```python
from build123d import *

# Parameters (mm, degrees)
SKETCH1_R                = 1.55
SKETCH1_R_2              = 7
SKETCH1_R_3              = 2.5
BOSS_EXTRUDE1_DEPTH      = 20
BOSS_EXTRUDE2_REACH      = 53.813
BOSS_EXTRUDE2_END_RADIUS = 18.9
BOSS_EXTRUDE3_REACH      = 55.526
BOSS_EXTRUDE3_END_RADIUS = 18.9
SKETCH3_W                = 6
SKETCH3_H                = 20
SKETCH5_R                = 1.675
CUT_EXTRUDE3_DEPTH       = 22.5
CUT_EXTRUDE4_DEPTH       = 11
CUT_EXTRUDE5_DEPTH       = 5.25
SKETCH8_R                = 1.06
CUT_EXTRUDE6_DEPTH       = 54.525694884
SKETCH9_R                = 3
CUT_EXTRUDE7_DEPTH       = 10
SKETCH11_R               = 11.2
CUT_EXTRUDE9_DEPTH       = 2.35
CUT_EXTRUDE8_DEPTH       = 6


with BuildPart() as part:
    # Sketch1 → Boss-Extrude1 (new body)
    with BuildSketch(Plane(origin=(0, 0, 0), x_dir=(1, 0, 0), z_dir=(0, 1, 0))):
        with BuildLine():
            Line((10.349494937, -15.814485593), (10.349494937, 8.416255239))
            ThreePointArc((10.349494937, 8.416255239), (10.822804202, 11.144484896), (8.349494937, 9.899494937))
            Line((8.349494937, 9.899494937), (8.349494937, -16.955705067))
            ThreePointArc((8.349494937, -16.955705067), (-17.76919177, 6.439396233), (17.273666667, 7.670100383))
            ThreePointArc((17.273666667, 7.670100383), (23, 0), (17.273666667, -7.670100383))
            ThreePointArc((17.273666667, -7.670100383), (14.399392933, -12.242037541), (10.349494937, -15.814485593))
        make_face()
        with Locations(Location((-9.899494937, 9.899494937, 0), (0, 0, 270))):
            Circle(SKETCH1_R, mode=Mode.SUBTRACT)
        with Locations(Location((-9.899494937, -9.899494937, 0), (0, 0, 270))):
            Circle(SKETCH1_R, mode=Mode.SUBTRACT)
        with Locations(Location((0, 0, 0), (0, 0, 270))):
            Circle(SKETCH1_R_2, mode=Mode.SUBTRACT)
        with Locations(Location((15, 0, 0), (0, 0, 270))):
            Circle(SKETCH1_R_3, mode=Mode.SUBTRACT)
    extrude(amount=BOSS_EXTRUDE1_DEPTH)

    # Boss-Extrude2: up to this cylinder (the profile starts outside it)
    boss_extrude2_end = Plane(origin=(0, 6.495191, 0), z_dir=(0, -1, 0)) * Cylinder(BOSS_EXTRUDE2_END_RADIUS, 146.426, mode=Mode.PRIVATE)
    # Sketch2 → Boss-Extrude2 (add, up to the surface)
    with BuildSketch(Plane.XY.offset(-23), mode=Mode.PRIVATE) as boss_extrude2_sk1:
        Polygon((14.1, 6.495190528), (10.35, 0), (2.85, 0), (-0.9, 6.495190528), (2.85, 12.990381057), (10.35, 12.990381057), align=None)
    boss_extrude2_tool1 = extrude(boss_extrude2_sk1.sketch, amount=BOSS_EXTRUDE2_REACH, mode=Mode.PRIVATE) - boss_extrude2_end
    add(boss_extrude2_tool1.solids().sort_by_distance((6.6, 6.495191, -23))[0])

    # Boss-Extrude3: up to this cylinder (the profile starts outside it)
    boss_extrude3_end = Plane(origin=(0, 9.928375, 0), z_dir=(0, -1, 0)) * Cylinder(BOSS_EXTRUDE3_END_RADIUS, 149.99525, mode=Mode.PRIVATE)
    # Sketch3 → Boss-Extrude3 (add, up to the surface)
    with BuildSketch(Plane.XY.offset(21), mode=Mode.PRIVATE) as boss_extrude3_sk1:
        with BuildLine():
            Line((8.349494937, 20), (3.349494937, 20))
            Line((3.349494937, 20), (3.349494937, 8.936698586))
            ThreePointArc((3.349494937, 8.936698586), (2.099494937, 6.5), (3.349494937, 4.063301414))
            Line((3.349494937, 4.063301414), (3.349494937, 0))
            Line((3.349494937, 0), (8.349494937, 0))
            Line((8.349494937, 0), (8.349494937, 20))
        make_face()
    boss_extrude3_tool1 = extrude(boss_extrude3_sk1.sketch, amount=-BOSS_EXTRUDE3_REACH, mode=Mode.PRIVATE) - boss_extrude3_end
    add(boss_extrude3_tool1.solids().sort_by_distance((5.726294, 9.85675, 21))[0])
    # Sketch3 → Boss-Extrude3 (add, up to the surface)
    with BuildSketch(Plane.XY.offset(21), mode=Mode.PRIVATE) as boss_extrude3_sk2:
        with Locations((13.349494937, 10)):
            Rectangle(SKETCH3_W, SKETCH3_H)
    boss_extrude3_tool2 = extrude(boss_extrude3_sk2.sketch, amount=-BOSS_EXTRUDE3_REACH, mode=Mode.PRIVATE) - boss_extrude3_end
    add(boss_extrude3_tool2.solids().sort_by_distance((13.349495, 10, 21))[0])

    # Sketch5 → Cut-Extrude3 (cut)
    with BuildSketch(Plane(origin=(16.349494937, 0, 0), x_dir=(0, 0, -1), z_dir=(1, 0, 0))):
        with Locations(Location((-17, 12, 0), (0, 0, 90))):
            Circle(SKETCH5_R)
    extrude(amount=-CUT_EXTRUDE3_DEPTH, mode=Mode.SUBTRACT)

    # Sketch6 → Cut-Extrude4 (cut)
    with BuildSketch(Plane(origin=(-6.150505063, 0, 0), x_dir=(0, 0, -1), z_dir=(1, 0, 0))):
        Polygon((-20.35, 12), (-18.675, 9.098814897), (-15.325, 9.098814897), (-13.65, 12), (-15.325, 14.901185103), (-18.675, 14.901185103), align=None)
    extrude(amount=CUT_EXTRUDE4_DEPTH, mode=Mode.SUBTRACT)

    # Sketch7 → Cut-Extrude5 (cut)
    with BuildSketch(Plane(origin=(0, 4.25, 0), x_dir=(1, 0, 0), z_dir=(0, 1, 0))):
        with BuildLine():
            Line((6.29798001, 4), (5.744562647, 4))
            Line((5.744562647, 4), (5.744562647, -4))
            Line((5.744562647, -4), (6.29798001, -4))
            ThreePointArc((6.29798001, -4), (24.577324882, 0), (6.29798001, 4))
        make_face()
    extrude(amount=CUT_EXTRUDE5_DEPTH, mode=Mode.SUBTRACT)

    # Sketch8 → Cut-Extrude6 (cut, through all)
    with BuildSketch(Plane(origin=(0, 0, -23), x_dir=(-1, 0, 0), z_dir=(0, 0, -1))):
        with Locations((-6.6, 6.495190528)):
            Circle(SKETCH8_R)
    extrude(amount=-CUT_EXTRUDE6_DEPTH, mode=Mode.SUBTRACT)

    # Sketch9 → Cut-Extrude7 (cut)
    with BuildSketch(Plane(origin=(0, 0, -23), x_dir=(-1, 0, 0), z_dir=(0, 0, -1))):
        with Locations((-6.6, 6.495190528)):
            Circle(SKETCH9_R)
    extrude(amount=-CUT_EXTRUDE7_DEPTH, mode=Mode.SUBTRACT)

    # Sketch11 → Cut-Extrude9 (cut)
    with BuildSketch(Plane(origin=(0, 20, 0), x_dir=(1, 0, 0), z_dir=(0, 1, 0))):
        Circle(SKETCH11_R)
    extrude(amount=-CUT_EXTRUDE9_DEPTH, mode=Mode.SUBTRACT)

    # Sketch10 → Cut-Extrude8 (cut)
    with BuildSketch(Plane(origin=(0, 20, 0), x_dir=(1, 0, 0), z_dir=(0, 1, 0))):
        Polygon((15, 4.7), (10.929680602, 2.35), (10.349494937, 2.35), (10.349494937, -2.35), (10.929680602, -2.35), (15, -4.7), (19.070319398, -2.35), (19.070319398, 2.35), align=None)
    extrude(amount=-CUT_EXTRUDE8_DEPTH, mode=Mode.SUBTRACT)

    # Cut-Revolve1: read off the stored shape, not the designer's step
    # Cut-Revolve1: loft between two sections, ruled curve by curve
    cut_revolve1_from = [
        Edge.make_three_point_arc((7.653578644, 6.608263478, -9.001288479), (6.491231459, 7.554083708, -9.001288479), (5.545411229, 6.391736522, -9.001288479)),
        Edge.make_three_point_arc((5.545411229, 6.391736522, -9.001288479), (6.707758415, 5.445916292, -9.001288479), (7.653578644, 6.608263478, -9.001288479)),
    ]
    cut_revolve1_to = [
        Edge.make_three_point_arc((9.086412031, 6.755427811, -4), (6.344067126, 8.986917094, -4), (4.112577842, 6.244572189, -4)),
        Edge.make_three_point_arc((4.112577842, 6.244572189, -4), (6.854922748, 4.013082906, -4), (9.086412031, 6.755427811, -4)),
    ]
    cut_revolve1 = Solid(Shell([*[Face.make_surface_from_curves(cut_revolve1_from[k], cut_revolve1_to[k]) for k in range(2)], Face(Wire(cut_revolve1_from)), Face(Wire(cut_revolve1_to))]))
    add(cut_revolve1, mode=Mode.SUBTRACT)


solid = part.part
```
Input: part model. Units: mm. Frame: model coordinates. A direction names the side the tool comes from. Round coordinates to 2 decimals unless told otherwise and drop trailing zeros. Loops run counter-clockwise (first coordinate to the right, second up) from the corner with the lowest first, then second, coordinate; pieces in that order, holes last. Notation, with made-up numbers: (-30, 36.25) -> (7, 36.25) arc R30 ccw to (7, 59.25) -> close; hole circle Ø8 at (-13.75, 4). An arc over 180 degrees is marked (long way). Write each question's results on one line, items separated by ' | '.
1. First-contact query: P1, Ø3, axis at x = -9.9, z = -9.9, coming from the +Y side; P2, Ø8, axis at x = -2.5, y = 8.5, coming from the +Z side; P3, Ø6, axis at y = 5, z = 3.5, coming from the -X side; P4, Ø1, axis at y = 12, z = -17, coming from the -X side. Flat tips, straight axial feed; report the tip coordinate or a pass-through.
Geometry results:
P1: through | P2: z = 18.9 | P3: x = -18.89 | P4: x = -9.22
2. Section B-B (x = 0). Return loops of the section in (y, z) (3 decimals).
Geometry results:
outline: (0, -18.9) -> (4.936, -18.9) -> (4.936, -23) -> (8.054, -23) -> (8.054, -18.9) -> (20, -18.9) -> (20, -11.2) -> (17.65, -11.2) -> (17.65, -7) -> (0, -7) -> close; (0, 7) -> (17.65, 7) -> (17.65, 11.2) -> (20, 11.2) -> (20, 18.9) -> (14.511, 18.9) -> (14.901, 18.675) -> (14.901, 15.325) -> (12, 13.65) -> (9.099, 15.325) -> (9.099, 18.675) -> (9.489, 18.9) -> (0, 18.9) -> close
3. Section A-A (z = 17). Return loops of the section in (x, y) (1 decimal), and give its area (3 significant figures).
Geometry results:
outline: (-8.3, 0) -> (8.3, 0) -> (8.3, 10.3) -> (4.8, 10.3) -> (4.8, 9.1) -> (-6.2, 9.1) -> (-6.2, 14.9) -> (4.8, 14.9) -> (4.8, 13.7) -> (8.3, 13.7) -> (8.3, 20) -> (-8.3, 20) -> close; (10.3, 0) -> (16.3, 0) -> (16.3, 10.3) -> (10.3, 10.3) -> close; (10.3, 13.7) -> (16.3, 13.7) -> (16.3, 20) -> (10.3, 20) -> close; hole circle Ø2.1 at (6.6, 6.5) | area: 353 mm2
4. Section D-D (x = 13.5). Return loops of the section in (y, z) (3 decimals), and give its area (3 significant figures).
Geometry results:
outline: (0, -13.227) -> (5.456, -13.227) -> (5.456, -23) -> (7.534, -23) -> (7.534, -13.227) -> (20, -13.227) -> (20, -3.834) -> (14, -3.834) -> (14, -2) -> (9.5, -2) -> (9.5, -9.459) -> (4.25, -9.459) -> (4.25, -2) -> (0, -2) -> close; (0, 2) -> (4.25, 2) -> (4.25, 9.459) -> (9.5, 9.459) -> (9.5, 2) -> (14, 2) -> (14, 3.834) -> (20, 3.834) -> (20, 21) -> (0, 21) -> close; hole circle Ø3.35 at (12, 17) | area: 516 mm2
5. Section C-C (z = 0). State how many separate pieces and enclosed holes the cut face has, and give its area (3 significant figures).
Geometry results:
separate pieces: 7 | enclosed holes: 0 | area: 335 mm2
6. Ray query, line 1 (X direction, y = 10, z = 19.5); line 2 (Y direction, x = 15, z = -4); line 3 (Y direction, x = 6.6, z = -11.65). Return the intervals inside material, ascending. Write a range as from..to.
Geometry results:
line 1: 3.35..8.35, 10.35..16.35 | line 2: 0..4.25, 9.5..14 | line 3: 0..5.44, 7.56..20
7. Mould query, pull axis X, two halves, no side actions, for faces 6 (the face through (6, 20, 10)), 7 (the face through (7.25, 3.567, -18.07)), 8 (the face through (16.349, 10, 15)). Classes: +X half, -X half, draft (parallel to the pull), parting line (faces both ways), or undercut.
Geometry results:
face 6: draft | face 7: undercut | face 8: +X half
8. Set-up query: faces 1 (the face through (13.302, 6.838, -9.426)), 2 (the face through (7.94, 8.03, -6.47)), 3 (the face through (8.349, 10, 6)), 4 (the face through (5, 7, -13)), 5 (the face through (19.07, 17, 0)). Return all of +Z, -Z, +X, -X, +Y, -Y with unobstructed straight access to the full face (end or side cutting, diameter ignored); none if empty.
Geometry results:
face 1: none | face 2: +X | face 3: +Z, +Y, -Y | face 4: -Z | face 5: +Y
